Check sheet for the modelled part. Datum: model origin and axes. Units: mm. A direction names the side the tool comes from. Coordinates: 2 decimals unless noted, no trailing zeros. Loops run counter-clockwise (first coordinate to the right, second up) from the corner with the lowest first, then second, coordinate; pieces in that order, holes last. Notation, with made-up numbers: (88, 73) - (101, 73) arc R19 ccw to (101, 98) - close; hole circle Ø10 at (18, -24). An arc over 180 degrees is marked (long way). Use a Markdown table: item, result. Add a question column.
1) Go/stop test with flat-tipped pins: P1, Ø1.8, axis at x = 12, y = 1.5, coming from the -Z side; P2, Ø1.4, axis at y = 0.5, z = -11.5, coming from the -X side; P3, Ø2, axis at x = 4, z = 2.5, coming from the -Y side. Record where each tip stops, or that it passes through.
2) Tool access check on faces 4 (the cylindrical face through (-16.93, 0.76, 9.4)), 5 (the flat face through (10, 2, -10)), 6 (the flat face through (0, 0, 0)). Record the directions out of +Z, -Z, +X, -X, +Y, -Y that give a thin tool (end or side, any length) a straight path to the whole face; none if there is none.
3) Sectioned sample at D-D, the plane z = -2.25. Enter the section's corners in (x, y).
4) Draft check along Y on faces 1 (the cylindrical face through (-5.226, -0.645, -13.634)), 2 (the flat face through (-7, 1.3, -11.3)), 3 (the cylindrical face through (0.22, 2.93, 9.4)). Enter one of: pulls with the +Y half, pulls with the -Y half, needs draft (parallel to the pull), parting line crosses it, or undercut.
5) Thickness scan on line 1 (X direction, y = -1.4, z = -10.5); line 2 (Y direction, x = 14.5, z = -5); line 3 (Z direction, x = -8.5, y = 1.2). Record the ranges inside material, lowest first.
6) Sectioned sample at A-A, the plane z = -11.5. State how many separate pieces and enclosed holes the cut face has, then the cut area to 3 significant figures.
7) Sectioned sample at C-C, the plane x = -12. Enter the section's corners in (y, z), then the cut area to 3 significant figures.
from build123d import *

# Parameters (mm, degrees)
SKETCH1_W           = 35
SKETCH1_H           = 20
BOSS_EXTRUDE1_DEPTH = 3.5
SKETCH3_R           = 1.5
BOSS_EXTRUDE2_DEPTH = 3.5
LPATTERN1_COUNT     = 4
LPATTERN1_PITCH     = 10.5
FILLET1_R           = 2


with BuildPart() as part:
    # Sketch1 → Boss-Extrude1 (new body)
    with BuildSketch(Plane(origin=(0, 0, 0), x_dir=(1, 0, 0), z_dir=(0, 1, 0))):
        Rectangle(SKETCH1_W, SKETCH1_H)
    extrude(amount=BOSS_EXTRUDE1_DEPTH)

    # Sketch3 → Boss-Extrude2 (add)
    with BuildSketch(Plane(origin=(17.5, 0, 0), x_dir=(0, 0, -1), z_dir=(1, 0, 0))):
        with BuildLine():
            ThreePointArc((13.220333212, 1.958519537), (13.418028169, -1.993351189), (10, 0))
            Line((10, 0), (10, 3.5))
            Line((10, 3.5), (13.220333212, 1.958519537))
        make_face()
        with Locations((12.248880815, -0.070958288)):
            Circle(SKETCH3_R, mode=Mode.SUBTRACT)
    boss_extrude2 = extrude(amount=-BOSS_EXTRUDE2_DEPTH)

    # LPattern1: Boss-Extrude2 ×4
    with Locations(*[(-i * LPATTERN1_PITCH, 0, 0) for i in range(1, LPATTERN1_COUNT)]):
        add(boss_extrude2)

    # Fillet1
    fillet1_edges = [part.edges().sort_by_distance(p)[0] for p in [
        (17.5, 3.5, 0),
        (0, 3.5, 10),
        (-17.5, 3.5, 0),
        (-17.5, 1.75, 10),
        (17.5, 1.75, 10),
    ]]
    fillet(fillet1_edges, radius=FILLET1_R)


solid = part.part
Solved:
| question | item | result |
|---|---|---|
| 1 | P1 | stops at z = -10 |
| 1 | P2 | stops at x = -17.5 |
| 1 | P3 | stops at y = 0 |
| 2 | face 4 | +Z, -X, +Y, -Y |
| 2 | face 5 | -Z, +Y, -Y |
| 2 | face 6 | +Z, +X, -X, -Y |
| 3 | outline | (-17.5, 0) - (17.5, 0) - (17.5, 1.5) arc R2 ccw to (15.5, 3.5) - (-15.5, 3.5) arc R2 ccw to (-17.5, 1.5) - close |
| 4 | face 1 | undercut |
| 4 | face 2 | needs draft |
| 4 | face 3 | pulls with the +Y half |
| 5 | line 1 | x = -17.5 to -14, -7 to -3.5, 3.5 to 7, 14 to 17.5 |
| 5 | line 2 | y = 0 to 3.5 |
| 5 | line 3 | z = -10 to 10 |
| 6 | separate pieces | 8 |
| 6 | enclosed holes | 0 |
| 6 | area | 32.9 mm2 |
| 7 | outline | (0, -10) - (3.5, -10) - (3.5, 8) arc R2 ccw to (1.5, 10) - (0, 10) - close |
| 7 | area | 69.1 mm2 |
